from build123d import *

# Parameters (mm, degrees)
F0_R     = 1.5
F1_DEPTH = 3.175


# Not quite as in the source:
# - a length typed as a fraction of an inch, garbled in the dataset ("3 / 203.2 mm" for 3/8 in), is restored
# - a feature names something its author has since deleted; it is built from what else it names


with BuildPart() as f1:
    # F0 (on Top) → F1 (new body)
    with BuildSketch(Plane.XY):
        with BuildLine():
            ThreePointArc((-33.3848889083, 26.7107070004), (-34.5564617835, 29.5391341252), (-37.3848889083, 30.7107070004))
            ThreePointArc((-37.3848889083, 30.7107070004), (-41.3848889083, 26.7107070004), (-37.3848889083, 22.7107070004))
            ThreePointArc((-37.3848889083, 22.7107070004), (-34.5564617835, 23.8822798757), (-33.3848889083, 26.7107070004))
        make_face()
        with Locations((-37.3848889083, 26.7107070004)):
            Circle(F0_R, mode=Mode.SUBTRACT)
        with BuildLine():
            Line((-3.4348889083, 20.3883182257), (-16.1348889083, 20.3883182257))
            Line((-16.1348889083, 20.3883182257), (-16.1348889083, 31.8183182257))
            Line((-16.1348889083, 31.8183182257), (-16.1348889083, 39.4383182257))
            Line((-16.1348889083, 39.4383182257), (-16.1348889083, 51.9607070004))
            ThreePointArc((-16.1348889083, 51.9607070004), (-22.3588698081, 36.9346879002), (-37.3848889083, 30.7107070004))
            ThreePointArc((-37.3848889083, 30.7107070004), (-34.5564617835, 29.5391341252), (-33.3848889083, 26.7107070004))
            ThreePointArc((-33.3848889083, 26.7107070004), (-34.5564617835, 23.8822798757), (-37.3848889083, 22.7107070004))
            ThreePointArc((-37.3848889083, 22.7107070004), (-31.3137586061, 21.7575229445), (-25.8268376377, 18.9896932393))
            ThreePointArc((-25.8268376377, 18.9896932393), (-25.3822585347, 24.9465327374), (-20.2848889083, 21.8323056621))
            ThreePointArc((-20.2848889083, 21.8323056621), (-20.5921773878, 20.3982229772), (-21.4600849924, 19.215955771))
            ThreePointArc((-21.4600849924, 19.215955771), (-20.8930268384, 19.5596143827), (-20.2408664312, 19.6793766243))
            Line((-20.2408664312, 19.6793766243), (0.6710886146, 19.6793766243))
            ThreePointArc((0.6710886146, 19.6793766243), (1.3232490219, 19.5596143827), (1.8903071759, 19.215955771))
            ThreePointArc((1.8903071759, 19.215955771), (2.7810284068, 25.0250171826), (7.7151110917, 21.8323056621))
            ThreePointArc((7.7151110917, 21.8323056621), (7.329338167, 20.2349360357), (6.2570598212, 18.9896932393))
            ThreePointArc((6.2570598212, 18.9896932393), (11.7439807896, 21.7575229445), (17.8151110917, 22.7107070004))
            ThreePointArc((17.8151110917, 22.7107070004), (13.8151110917, 26.7107070004), (17.8151110917, 30.7107070004))
            ThreePointArc((17.8151110917, 30.7107070004), (2.7890919915, 36.9346879002), (-3.4348889083, 51.9607070004))
            Line((-3.4348889083, 51.9607070004), (-3.4348889083, 39.4383182257))
            Line((-3.4348889083, 39.4383182257), (-3.4348889083, 31.8183182257))
            Line((-3.4348889083, 31.8183182257), (-3.4348889083, 20.3883182257))
        make_face()
        Polygon((-16.1348889083, 31.8183182257), (-16.1348889083, 20.3883182257), (-3.4348889083, 20.3883182257), (-3.4348889083, 31.8183182257), (-6.6098889083, 31.8183182257), (-6.6098889083, 39.4383182257), (-3.4348889083, 39.4383182257), (-3.4348889083, 51.9607070004), (-3.4348889083, 83.8883182257), (-6.6098889083, 83.8883182257), (-6.6098889083, 109.2883182257), (-3.4348889083, 109.2883182257), (-3.4348889083, 134.6883182257), (-6.6098889083, 134.6883182257), (-6.6098889083, 160.0883182257), (-3.4348889083, 160.0883182257), (-3.4348889083, 185.4883182257), (-6.6098889083, 185.4883182257), (-6.6098889083, 210.8883182257), (-3.4348889083, 210.8883182257), (-3.4348889083, 236.2883182257), (-6.6098889083, 236.2883182257), (-6.6098889083, 261.6883182257), (-3.4348889083, 261.6883182257), (-3.4348889083, 274.3883182257), (-16.1348889083, 274.3883182257), (-16.1348889083, 261.6883182257), (-12.9598889083, 261.6883182257), (-12.9598889083, 236.2883182257), (-16.1348889083, 236.2883182257), (-16.1348889083, 210.8883182257), (-12.9598889083, 210.8883182257), (-12.9598889083, 185.4883182257), (-16.1348889083, 185.4883182257), (-16.1348889083, 160.0883182257), (-12.9598889083, 160.0883182257), (-12.9598889083, 134.6883182257), (-16.1348889083, 134.6883182257), (-16.1348889083, 109.2883182257), (-12.9598889083, 109.2883182257), (-12.9598889083, 83.8883182257), (-16.1348889083, 83.8883182257), (-16.1348889083, 51.9607070004), (-16.1348889083, 39.4383182257), (-12.9598889083, 39.4383182257), (-12.9598889083, 31.8183182257), align=None)
        with BuildLine():
            ThreePointArc((21.8151110917, 26.7107070004), (20.6435382165, 29.5391341252), (17.8151110917, 30.7107070004))
            ThreePointArc((17.8151110917, 30.7107070004), (13.8151110917, 26.7107070004), (17.8151110917, 22.7107070004))
            ThreePointArc((17.8151110917, 22.7107070004), (20.6435382165, 23.8822798757), (21.8151110917, 26.7107070004))
        make_face()
        with Locations((17.8151110917, 26.7107070004)):
            Circle(F0_R, mode=Mode.SUBTRACT)
        with BuildLine():
            ThreePointArc((-20.2848889083, 21.8323056621), (-25.3822585347, 24.9465327374), (-25.8268376377, 18.9896932393))
            ThreePointArc((-25.8268376377, 18.9896932393), (-23.6037799702, 18.3369945812), (-21.4600849924, 19.215955771))
            ThreePointArc((-21.4600849924, 19.215955771), (-20.5921773878, 20.3982229772), (-20.2848889083, 21.8323056621))
        make_face()
        with Locations((-23.7848889083, 21.8323056621)):
            Circle(F0_R, mode=Mode.SUBTRACT)
        with BuildLine():
            ThreePointArc((1.8903071759, 19.215955771), (4.0340021537, 18.3369945812), (6.2570598212, 18.9896932393))
            ThreePointArc((6.2570598212, 18.9896932393), (7.329338167, 20.2349360357), (7.7151110917, 21.8323056621))
            ThreePointArc((7.7151110917, 21.8323056621), (2.7810284068, 25.0250171826), (1.8903071759, 19.215955771))
        make_face()
        with Locations((4.2151110917, 21.8323056621)):
            Circle(F0_R, mode=Mode.SUBTRACT)
    extrude(amount=F1_DEPTH)


solid = f1.part
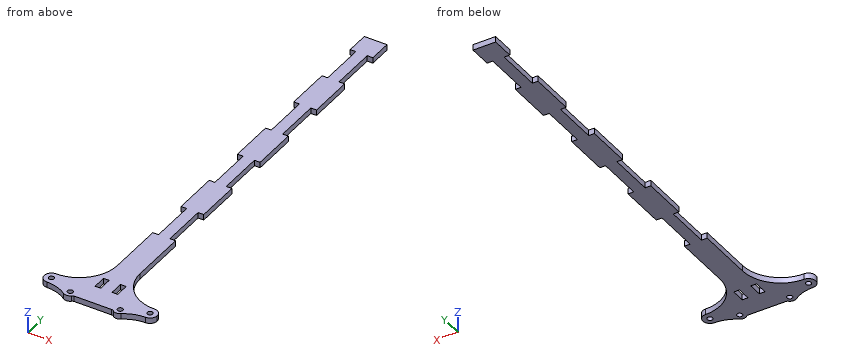
Input: part model. Units: mm. Frame: model coordinates. Coordinates: 2 decimals unless noted, no trailing zeros. Loops run counter-clockwise (first coordinate to the right, second up) from the corner with the lowest first, then second, coordinate; pieces in that order, holes last. Notation, with made-up numbers: (6.5, 0.5) -> (35.5, 0.5) arc R33 cw to (35.5, 39.5) -> close; hole circle Ø7 at (-20, 52.5). An arc over 180 degrees is marked (long way). Write item = value, one per line. Start each with the question number.
Item 1: Material intervals for line 1 (Y direction, x = -6.5, z = 1.9); line 2 (X direction, y = 165, z = 1); line 3 (X direction, y = 89.5, z = 1.3), sorted ascending.
Item 2: Cut plane B-B, the plane z = 2.65. Count the separate pieces of the cut face and the enclosed holes in it, plus the area to 3 significant figures.
Item 3: Cut plane A-A, the plane y = 35. Return loops of the section in (x, z) (3 decimals), plus the area to 3 significant figures.
Item 4: Cut plane C-C, the plane x = 11.5. Return loops of the section in (y, z) (3 decimals).
Item 5: First-contact query: P1, Ø1.6, axis at x = -14.5, z = 1, coming from the -Y side; P2, Ø1.6, axis at y = 177, z = 1.5, coming from the -X side; P3, Ø1, axis at y = 136.5, z = 1.5, coming from the +X side. Flat tips, straight axial feed; report the tip coordinate or a pass-through.
Item 6: Cut plane D-D, the plane y = 240. Return loops of the section in (x, z) (3 decimals), plus the area to 3 significant figures.
Ans:
q1.line_1 = 19.68 to 31.82, 39.44 to 83.89, 109.29 to 134.69, 160.09 to 185.49, 210.89 to 236.29, 261.69 to 274.39
q1.line_2 = -16.13 to -3.43
q1.line_3 = -12.96 to -6.61
q2.separate_pieces = 1
q2.enclosed_holes = 6
q2.area = 3,190 mm²
q3.outline = (-24.583, 0) -> (-16.135, 0) -> (-16.135, 3.175) -> (-24.583, 3.175) -> close; (-12.96, 0) -> (-6.61, 0) -> (-6.61, 3.175) -> (-12.96, 3.175) -> close; (-3.435, 0) -> (5.013, 0) -> (5.013, 3.175) -> (-3.435, 3.175) -> close
q3.area = 73.8 mm²
q4.outline = (21.677, 0) -> (31.671, 0) -> (31.671, 3.175) -> (21.677, 3.175) -> close
q5.P1 = 19.68
q5.P2 = -16.13
q5.P3 = -6.61
q6.outline = (-12.96, 0) -> (-6.61, 0) -> (-6.61, 3.175) -> (-12.96, 3.175) -> close
q6.area = 20.2 mm²
